from build123d import *

# Parameters (mm, degrees)
F0_W      = 50
F0_H      = 22
F1_DEPTH  = 12.5
F2_W      = 45
F2_H      = 15
F3_DEPTH  = 15
F4_R      = 2.5
F5_DEPTH  = 3
F6_R      = 2.5
F7_DEPTH  = 3
F8_R      = 2.5
F9_DEPTH  = 3
F10_R     = 2.5
F11_DEPTH = 3
F12_R     = 10
F13_DEPTH = 2
F14_R     = 10
F15_DEPTH = 2
F16_R     = 10
F17_DEPTH = 2
F18_R     = 10.0146932226
F19_DEPTH = 2
F20_R     = 7.5
F21_DEPTH = 1
F22_R     = 7.5
F23_DEPTH = 1
F24_R     = 7.5
F25_DEPTH = 1
F26_R     = 7.3021705666
F27_DEPTH = 1
F28_R     = 2.5
F29_DEPTH = 2
F30_R     = 2.5
F31_DEPTH = 2
F32_R     = 2.5
F33_DEPTH = 2
F34_R     = 2.5
F35_DEPTH = 2
F36_R     = 6
F37_DEPTH = 4
F38_R     = 6
F39_DEPTH = 4
F42_SIZE  = 7
F43_SIZE  = 7


# Not quite as in the source:
# - a pattern or mirror of a feature is missing from the dataset's text; its kind, count and spacing are read off the source's solid


with BuildPart() as f1:
    # F0 (on Front) → F1 (new body, symmetric)
    with BuildSketch(Plane.XZ):
        Rectangle(F0_W, F0_H)
    extrude(amount=F1_DEPTH, both=True)

    # F2 (on face) → F3 (join)
    with BuildSketch(Plane(origin=(0, 0, -11), x_dir=(1, 0, 0), z_dir=(0, 0, -1))):
        Rectangle(F2_W, F2_H)
    extrude(amount=F3_DEPTH)

    # F4 (on face) → F5 (join)
    with BuildSketch(Plane.XZ.offset(7.5)):
        with Locations((13.9349065721, -22.4036108702)):
            Circle(F4_R)
    extrude(amount=F5_DEPTH)

    # F6 (on face) → F7 (join)
    with BuildSketch(Plane.XZ.offset(7.5)):
        with Locations((-14.7780319676, -22.1367031336)):
            Circle(F6_R)
    extrude(amount=F7_DEPTH)

    # F8 (on face) → F9 (join)
    with BuildSketch(Plane(origin=(0, 7.5, 0), x_dir=(-1, 0, 0), z_dir=(0, 1, 0))):
        with Locations((14.7414254025, -22.1880879253)):
            Circle(F8_R)
    extrude(amount=F9_DEPTH)

    # F10 (on face) → F11 (join)
    with BuildSketch(Plane(origin=(0, 7.5, 0), x_dir=(-1, 0, 0), z_dir=(0, 1, 0))):
        with Locations((-13.9084318653, -22.4365219474)):
            Circle(F10_R)
    extrude(amount=F11_DEPTH)

    # F12 (on face) → F13 (join)
    with BuildSketch(Plane(origin=(0, 10.5, 0), x_dir=(-1, 0, 0), z_dir=(0, 1, 0))):
        with Locations((-13.9084318653, -22.4365219474)):
            Circle(F12_R)
    extrude(amount=F13_DEPTH)

    # F14 (on face) → F15 (join)
    with BuildSketch(Plane(origin=(0, 10.5, 0), x_dir=(-1, 0, 0), z_dir=(0, 1, 0))):
        with Locations((14.7414254025, -22.1880879253)):
            Circle(F14_R)
    extrude(amount=F15_DEPTH)

    # F16 (on face) → F17 (join)
    with BuildSketch(Plane.XZ.offset(10.5)):
        with Locations((-14.7780319676, -22.1367031336)):
            Circle(F16_R)
    extrude(amount=F17_DEPTH)

    # F18 (on face) → F19 (join)
    with BuildSketch(Plane.XZ.offset(10.5)):
        with Locations((13.9349065721, -22.4036108702)):
            Circle(F18_R)
    extrude(amount=F19_DEPTH)

    # F20 (on face) → F21 (join)
    with BuildSketch(Plane.XZ.offset(12.5)):
        with Locations((-14.7780319676, -22.1367031336)):
            Circle(F20_R)
    extrude(amount=F21_DEPTH)

    # F22 (on face) → F23 (join)
    with BuildSketch(Plane.XZ.offset(12.5)):
        with Locations((13.9349065721, -22.4036108702)):
            Circle(F22_R)
    extrude(amount=F23_DEPTH)

    # F24 (on face) → F25 (join)
    with BuildSketch(Plane(origin=(0, 12.5, 0), x_dir=(-1, 0, 0), z_dir=(0, 1, 0))):
        with Locations((-13.9084318653, -22.4365219474)):
            Circle(F24_R)
    extrude(amount=F25_DEPTH)

    # F26 (on face) → F27 (join)
    with BuildSketch(Plane(origin=(0, 12.5, 0), x_dir=(-1, 0, 0), z_dir=(0, 1, 0))):
        with Locations((14.7414254025, -22.1880879253)):
            Circle(F26_R)
    extrude(amount=F27_DEPTH)

    # F28 (on face) → F29 (join)
    with BuildSketch(Plane(origin=(0, 13.5, 0), x_dir=(-1, 0, 0), z_dir=(0, 1, 0))):
        with Locations((-13.9084318653, -22.4365219474)):
            Circle(F28_R)
    extrude(amount=F29_DEPTH)

    # F30 (on face) → F31 (join)
    with BuildSketch(Plane(origin=(0, 13.5, 0), x_dir=(-1, 0, 0), z_dir=(0, 1, 0))):
        with Locations((14.7414254025, -22.1880879253)):
            Circle(F30_R)
    extrude(amount=F31_DEPTH)

    # F32 (on face) → F33 (join)
    with BuildSketch(Plane.XZ.offset(13.5)):
        with Locations((-14.7780319676, -22.1367031336)):
            Circle(F32_R)
    extrude(amount=F33_DEPTH)

    # F34 (on face) → F35 (join)
    with BuildSketch(Plane.XZ.offset(13.5)):
        with Locations((13.9349065721, -22.4036108702)):
            Circle(F34_R)
    extrude(amount=F35_DEPTH)

    # F36 (on face) → F37 (join)
    with BuildSketch(Plane(origin=(-22.5, 0, 0), x_dir=(0, -1, 0), z_dir=(-1, 0, 0))):
        with Locations((0, -18.4352861294)):
            Circle(F36_R)
    extrude(amount=F37_DEPTH)

    # F38 (on face) → F39 (join)
    with BuildSketch(Plane.YZ.offset(22.5)):
        with Locations((0, -18.4992050543)):
            Circle(F38_R)
    extrude(amount=F39_DEPTH)

    # F40 (on face) → F41 (revolve)
    with BuildSketch(Plane(origin=(-26.5, 0, 0), x_dir=(0, -1, 0), z_dir=(-1, 0, 0))):
        with BuildLine():
            Line((0, -23.4352861294), (0, -13.4352861294))
            ThreePointArc((0, -13.4352861294), (-5, -18.4352861294), (0, -23.4352861294))
        make_face()
    f41 = revolve(axis=Axis((-26.5, 0, -18.4352861294), (0, 0, -1)))

    # F41_copies: F41 across plane
    add(f41.mirror(Plane(origin=(0, 0, 0), x_dir=(0, 0, 1), z_dir=(1, 0, 0))))

    # F42
    f42_edges = [f1.edges().sort_by_distance(p)[0] for p in [
        (-25, 0, 11),
    ]]
    chamfer(f42_edges, length=F42_SIZE)

    # F43
    f43_edges = [f1.edges().sort_by_distance(p)[0] for p in [
        (25, 0, 11),
    ]]
    chamfer(f43_edges, length=F43_SIZE)


solid = f1.part
Design review of the part built by this model. Coordinates are the model's own, in mm. A direction names the side the tool comes from. Coordinates: 2 decimals unless noted, no trailing zeros. Order: outer loops, then holes, each group sorted by start corner. A loop starts at its lowest first (then second) coordinate and runs counter-clockwise, first axis right, second up. Notation, with made-up numbers: (44, 12.25) -> (89, 12.25) arc R8 cw to (89, 21.25) -> close; hole circle Ø6 at (-13.5, 35.5). An arc over 180 degrees is marked (long way). Use one line per item in the form item = value. Start each with the question number.
(1) Insertion check: pin 1 (12 mm diameter, centred on y = -1, z = 0.5, fed in from -X); pin 2 (4.5 mm diameter, centred on x = 7.5, y = -2.5, fed in from -Z); pin 3 (2 mm diameter, centred on y = -2, z = -16.5, fed in from +X); pin 4 (3 mm diameter, centred on y = 6, z = -28, fed in from -X). Each pin has a flat end and moves straight along its axis. Give the tip position at first contact, or say it passes through.
(2) For probe 1 along Y at (x, z) = (-13, -27); probe 2 along Y at (x, z) = (11, -21); probe 3 along Y at (x, z) = (4, -20.5), list the stretches that pass through material, from the lowest coordinate up.
(3) Add section B-B on y = 0. State the section outline as (x, z) points.
(4) Add section A-A on x = -6.5. State the section outline as (y, z) points.
(5) Add section C-C on z = 6. State the section outline as (x, y) points, plus the area to 3 significant figures.
(6) Add section D-D on y = 3.5. State the section outline as (x, z) points, plus the area to 3 significant figures.
(7) For faces 5 (the flat face through (26.5, -4, -15)), 6 (the flat face through (0, -12.5, 0)), 7 (the cylindrical face through (-10.164, -11.486, -31.008)), 8 (the cylindrical face through (11.524, 14.486, -21.686)), 9 (the flat face through (0, -7.5, -18)), list the 3-axis set-ups (+Z, -Z, +X, -X, +Y, -Y) from which the entire face can be reached by the end or side of a thin tool; tool diameter is ignored.
(8) The part is to be moulded in two halves that separate along Y. For faces 1 (the cylindrical face through (-21.706, 12.993, -19.995)), 2 (the flat face through (0, 0, -26)), 3 (the cylindrical face through (-16.621, -8.979, -20.447)), 4 (the flat face through (-18, 13.5, -22)), say which applies: +Y half, -Y half, draft (parallel to the pull), parting line (faces both ways), or undercut.
Answer block:
q1.pin_1 = -25
q1.pin_2 = -26
q1.pin_3 = 31.17
q1.pin_4 = through
q2.probe_1 = -13.5 to -10.5, 10.5 to 13.5
q2.probe_2 = -13.5 to -10.5, -7.5 to 7.5, 10.5 to 13.5
q2.probe_3 = -7.5 to 7.5
q3.outline = (-26.5, -24.44) -> (-22.5, -24.44) -> (-22.5, -26) -> (22.5, -26) -> (22.5, -24.5) -> (26.5, -24.5) -> (26.5, -23.44) arc R5 ccw to (26.5, -13.44) -> (26.5, -12.5) -> (22.5, -12.5) -> (22.5, -11) -> (25, -11) -> (25, 4) -> (18, 11) -> (-18, 11) -> (-25, 4) -> (-25, -11) -> (-22.5, -11) -> (-22.5, -12.44) -> (-26.5, -12.44) -> (-26.5, -13.44) arc R5 ccw to (-26.5, -23.44) -> close
q4.outline = (-12.5, -27.75) -> (-10.5, -27.75) -> (-10.5, -16.53) -> (-12.5, -16.53) -> close; (-12.5, -11) -> (-7.5, -11) -> (-7.5, -26) -> (7.5, -26) -> (7.5, -11) -> (12.5, -11) -> (12.5, 11) -> (-12.5, 11) -> close; (10.5, -27.85) -> (12.5, -27.85) -> (12.5, -16.52) -> (10.5, -16.52) -> close
q5.outline = (-23, -12.5) -> (23, -12.5) -> (23, 12.5) -> (-23, 12.5) -> close
q5.area = 1,150 mm²
q6.outline = (-26.5, -23.31) -> (-22.5, -23.31) -> (-22.5, -26) -> (22.5, -26) -> (22.5, -23.37) -> (26.5, -23.37) -> (26.5, -22.01) arc R3.57 ccw to (26.5, -14.86) -> (26.5, -13.63) -> (22.5, -13.63) -> (22.5, -11) -> (25, -11) -> (25, 4) -> (18, 11) -> (-18, 11) -> (-25, 4) -> (-25, -11) -> (-22.5, -11) -> (-22.5, -13.56) -> (-26.5, -13.56) -> (-26.5, -14.86) arc R3.57 ccw to (-26.5, -22.01) -> close
q6.area = 1,840 mm²
q7.face_5 = +X
q7.face_6 = +Z, +X, -X, -Y
q7.face_7 = -Y
q7.face_8 = +Y
q7.face_9 = none
q8.face_1 = draft
q8.face_2 = undercut
q8.face_3 = undercut
q8.face_4 = +Y half
